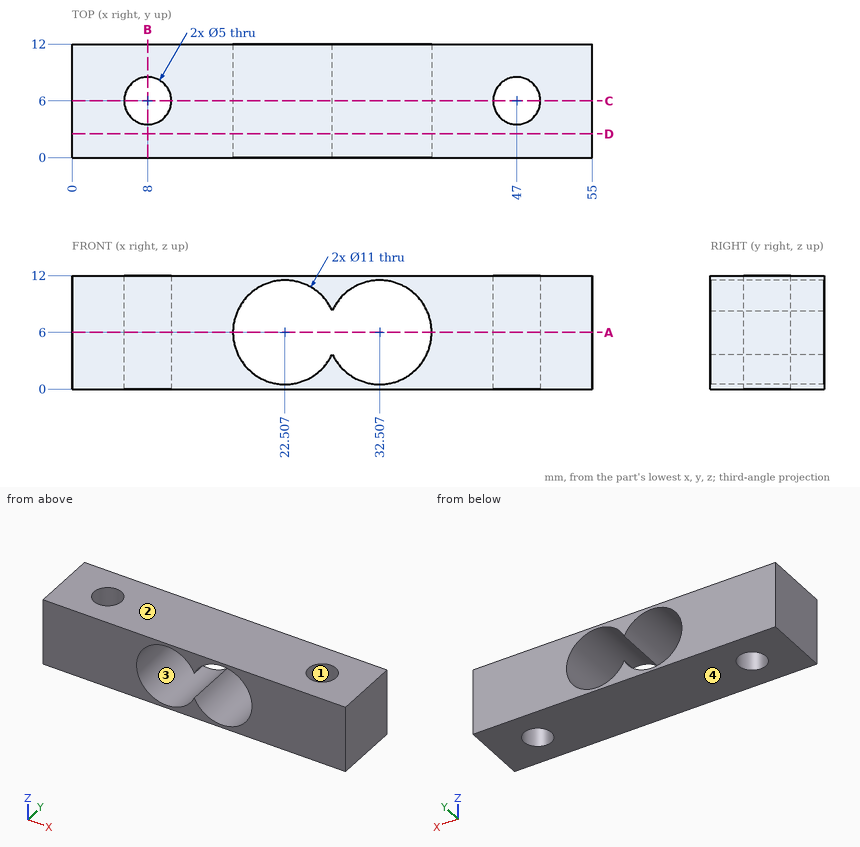
Geometry: see drawing. Coordinates: mm, zero at the bounding-box minimum. Give positions to 0.01 mm unless a question says otherwise; leave off trailing zeros. Loops run counter-clockwise (first coordinate to the right, second up) from the corner with the lowest first, then second, coordinate; pieces in that order, holes last. Notation, with made-up numbers: (87.5, 16) -> (100.5, 16) arc R28 cw to (100.5, 50) -> close; hole circle Ø8 at (66, 52.5). An arc over 180 degrees is marked (long way). Put each result on its own line as item: value.
1. Cut plane C-C (y = 6). Return the cut outline in (x, z).
Taken from the geometry:
outline: (0, 0) -> (5.5, 0) -> (5.5, 12) -> (0, 12) -> close; (10.5, 0) -> (44.5, 0) -> (44.5, 12) -> (10.5, 12) -> close; (49.5, 0) -> (55, 0) -> (55, 12) -> (49.5, 12) -> close; hole (27.51, 3.71) arc R5.5 ccw (long way) to (27.51, 8.29) arc R5.5 ccw (long way) to start
2. Pin query (flat end, axial travel): P1, Ø1.5, axis at x = 18, z = 6.5, coming from the +Y side. Return the tip coordinate at first contact, or that it passes through.
Taken from the geometry:
P1: passes through
3. Cut plane B-B (x = 8). Return the cut outline in (y, z).
Taken from the geometry:
outline: (0, 0) -> (3.5, 0) -> (3.5, 12) -> (0, 12) -> close; (8.5, 0) -> (12, 0) -> (12, 12) -> (8.5, 12) -> close
4. Cut plane A-A (z = 6). Return the cut outline in (x, y).
Taken from the geometry:
outline: (0, 0) -> (17.01, 0) -> (17.01, 12) -> (0, 12) -> close; (38.01, 0) -> (55, 0) -> (55, 12) -> (38.01, 12) -> close; hole circle Ø5 at (8, 6); hole circle Ø5 at (47, 6)
5. Pull-direction query (Z, two-part tool) for the marked faces 1, 2, 3 and 4; classes: released by +Z, released by -Z, zero draft, split by the parting line, or undercut.
Taken from the geometry:
face 1: zero draft
face 2: released by +Z
face 3: undercut
face 4: released by -Z
6. Cut plane D-D (y = 2.5). Return the cut outline in (x, z).
Taken from the geometry:
outline: (0, 0) -> (55, 0) -> (55, 12) -> (0, 12) -> close; hole (27.51, 3.71) arc R5.5 ccw (long way) to (27.51, 8.29) arc R5.5 ccw (long way) to start
7. Ray query, line 1 along Y through (x, z) = (8, 6.5); line 2 along X through (y, z) = (1.25, 2.5); line 3 along X through (y, z) = (2.5, 9.25). Return the intervals inside material, ascending. Write a range as [from, to].
Taken from the geometry:
line 1: y = [0, 3.5], [8.5, 12]
line 2: x = [0, 18.26], [26.75, 28.26], [36.75, 55]
line 3: x = [0, 18.07], [26.94, 28.07], [36.94, 55]
